Work out the finished part from the listing and answer in its coordinate system (mm). Give positions to 0.01 mm unless a question says otherwise; leave off trailing zeros. Write each loop counter-clockwise with the first axis right and the second up, starting at its lowest first coordinate (ties: lowest second). Pieces come first, ordered by that corner, then holes. Notation, with made-up numbers: (-20.75, 15.5) -> (35.25, 15.5) arc R21 ccw to (35.25, 28.5) -> close; hole circle Ø4 at (32, -6.75). An arc over 180 degrees is marked (long way). Write item = value, one per line. Start each with the question number.
from build123d import *

# Parameters (mm, degrees)
F0_W     = 5
F0_H     = 5
F2_D     = 3
F2_DEPTH = 95.001
F3_D     = 3


with BuildPart() as f1:
    # F0 (on Front) → F1 (revolve)
    with BuildSketch(Plane.XZ):
        with Locations((-92.5, 2.5)):
            Rectangle(F0_W, F0_H)
    revolve(axis=Axis((0, 0, 1.25), (0, 0, 1)))

    # F2 (through all, one way)
    with BuildSketch(Plane.XZ):
        with Locations((0, 2.5)):
            Circle(F2_D / 2)
    extrude(amount=-F2_DEPTH, mode=Mode.SUBTRACT)

    # F3 (through all)
    with Locations(Plane(origin=(0, 0, 0), x_dir=(1, 0, 0), z_dir=(0, 1, 0))):
        with Locations((0, -2.5)):
            Hole(F3_D / 2)


solid = f1.part
(1) A cutting plane is placed at B-B, the plane x = 83. Write down the section's boundary in (y, z), then the cut area to 3 significant figures.
(2) Find the intervals of material crossed by line 1 along Z through (x, y) = (0, -92); line 2 along X through (y, z) = (0, 3.35); line 3 along Y through (x, z) = (2, 2.2), in increasing order.
(3) Each of these flat-tipped pins is pushed along its axis until it touches: pin 1 (1 mm diameter, centred on y = -46.5, z = 1, fed in from +X); pin 2 (3 mm diameter, centred on y = -70.5, z = 3, fed in from -X). Where does it stop, or does it pass through?
(4) A cutting plane is placed at A-A, the plane y = 0. Write down the section's boundary in (x, z), then the cut area to 3 significant figures.
(5) Determine the mould class of faces 1 (the flat face through (-70, -57, 5)), 2 (the cylindrical face through (20.59, 92.74, 2.54)), 3 (the cylindrical face through (-41.53, 79.845, 2.535)) for opening direction Y: pulls with the +Y half, pulls with the -Y half, needs draft (parallel to the pull), parting line crosses it, or undercut.
Results list:
q1.outline = (-46.22, 0) -> (-34.8, 0) -> (-34.8, 5) -> (-46.22, 5) -> close; (34.8, 0) -> (46.22, 0) -> (46.22, 5) -> (34.8, 5) -> close
q1.area = 114 mm²
q2.line_1 = 0 to 1, 4 to 5
q2.line_2 = -95 to -90, 90 to 95
q2.line_3 = -94.98 to -89.98, 89.98 to 94.98
q3.pin_1 = 83.12
q3.pin_2 = -65.3
q4.outline = (-95, 0) -> (-90, 0) -> (-90, 5) -> (-95, 5) -> close; (90, 0) -> (95, 0) -> (95, 5) -> (90, 5) -> close
q4.area = 50.0 mm²
q5.face_1 = needs draft
q5.face_2 = parting line crosses it
q5.face_3 = undercut
